Check sheet for the modelled part. Datum: model origin and axes. Units: mm. Face numbers are marked on the shaded views. A direction names the side the tool comes from. Coordinates: 2 decimals unless noted, no trailing zeros. Loops run counter-clockwise (first coordinate to the right, second up) from the corner with the lowest first, then second, coordinate; pieces in that order, holes last. Notation, with made-up numbers: M 52,-7.5 L 81,-7.5 A18 ccw 81,25.5 Z; hole C -33,65 d9. An arc over 180 degrees is marked long. Return JSON: item names as keys, results as strings.
from build123d import *

# Parameters (mm, degrees)
SKETCH1_R           = 9
BOSS_EXTRUDE1_DEPTH = 5
SKETCH2_R           = 3
SKETCH2_R_2         = 2
BOSS_EXTRUDE2_DEPTH = 6
CUT_EXTRUDE1_DEPTH  = 17.822603841
CUT_EXTRUDE2_DEPTH  = 3
CUT_EXTRUDE3_DEPTH  = 8


with BuildPart() as part:
    # Sketch1 → Boss-Extrude1 (new body)
    with BuildSketch(Plane.XY):
        Circle(SKETCH1_R)
    extrude(amount=BOSS_EXTRUDE1_DEPTH)

    # Sketch2 → Boss-Extrude2 (add)
    with BuildSketch(Plane.XY.offset(5)):
        Circle(SKETCH2_R)
        with Locations(Location((-7, 0, 0), (0, 0, 179.999350333))):
            Circle(SKETCH2_R_2)
    extrude(amount=BOSS_EXTRUDE2_DEPTH)

    # Sketch3 → Cut-Extrude1 (cut, through all)
    with BuildSketch(Plane.XY.offset(11)):
        Polygon((-1.616580754, 0), (-0.808290377, -1.4), (0.808290377, -1.4), (1.616580754, 0), (0.808290377, 1.4), (-0.808290377, 1.4), align=None)
    extrude(amount=-CUT_EXTRUDE1_DEPTH, mode=Mode.SUBTRACT)

    # Sketch4 → Cut-Extrude2 (cut)
    with BuildSketch(Plane(origin=(0, 0, 0), x_dir=(-1, 0, 0), z_dir=(0, 0, -1))):
        Polygon((-4.099186911, 0), (-2.049593456, -3.55), (2.049593456, -3.55), (4.099186911, 0), (2.049593456, 3.55), (-2.049593456, 3.55), align=None)
    extrude(amount=-CUT_EXTRUDE2_DEPTH, mode=Mode.SUBTRACT)

    # Sketch5 → Cut-Extrude3 (cut)
    with BuildSketch(Plane.XZ.offset(-3.55)):
        with BuildLine():
            Line((1, 1.756249669), (1, -1.040433474))
            Line((1, -1.040433474), (-1, -1.040433474))
            Line((-1, -1.040433474), (-1, 1.756249669))
            ThreePointArc((-1, 1.756249669), (0, 2.756249669), (1, 1.756249669))
        make_face()
    extrude(amount=-CUT_EXTRUDE3_DEPTH, mode=Mode.SUBTRACT)


solid = part.part
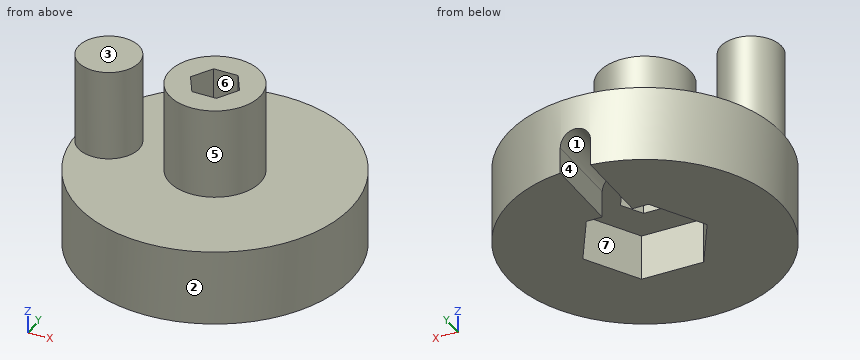
1) Scan lines: line 1 along Z through (x, y) = (3.5, -2); line 2 along Z through (x, y) = (-3.75, 0.5); line 3 along X through (y, z) = (1.5, 2). Record each from-to range of solid material in increasing order. Write a range as [from, to].
Answers:
{"line 1": "[0, 5]", "line 2": "[3, 5]", "line 3": "[-8.87, -3.23], [3.23, 8.87]"}
2) Go/stop test with flat-tipped pins: pin 1 Ø0.5 at (y, z) = (7, 0.5) entering from -X; pin 2 Ø1.4 at (y, z) = (5.5, 1) entering from +X; pin 3 Ø0.5 at (x, z) = (0, 6.5) entering from -Y; pin 4 Ø10 at (x, y) = (6.5, -1.5) entering from -Z. Record where each tip stops, or that it passes through.
Answers:
{"pin 1": "x = -5.95", "pin 2": "x = 7.61", "pin 3": "y = -3", "pin 4": "z = 0"}
3) Section check C-C on z = 3.25. Record the cut outline in (x, y), then the cut area to 3 significant figures.
Answers:
{"outline": "C 0,0 d18; hole M -1.62,0 L -0.81,-1.4 L 0.81,-1.4 L 1.62,0 L 0.81,1.4 L -0.81,1.4 Z", "area": "248 mm²"}
4) Section check B-B on x = 0. Record the cut outline in (y, z), then the cut area to 3 significant figures.
Answers:
{"outline": "M -9,0 L -3.55,0 L -3.55,3 L -1.4,3 L -1.4,11 L -3,11 L -3,5 L -9,5 Z; M 1.4,3 L 3.55,3 L 3.55,2.76 L 9,2.76 L 9,5 L 3,5 L 3,11 L 1.4,11 Z", "area": "67.3 mm²"}
5) Section check A-A on z = 7.5. Record the cut outline in (x, y), then the cut area to 3 significant figures.
Answers:
{"outline": "C -7,0 d4; C 0,0 d6; hole M -1.62,0 L -0.81,-1.4 L 0.81,-1.4 L 1.62,0 L 0.81,1.4 L -0.81,1.4 Z", "area": "34.1 mm²"}
6) Draft check along X on the marked faces 1, 2 and 3. Enter one of: +X half, -X half, draft (parallel to the pull), parting line (faces both ways), or undercut.
Answers:
{"face 1": "undercut", "face 2": "parting line", "face 3": "draft"}
7) Section check D-D on x = -7. Record the cut outline in (y, z), then the cut area to 3 significant figures.
Answers:
{"outline": "M -5.66,0 L 5.66,0 L 5.66,5 L 2,5 L 2,11 L -2,11 L -2,5 L -5.66,5 Z", "area": "80.6 mm²"}
8) Set-up check for the marked faces 4, 5, 6 and 7: record each of +Z, -Z, +X, -X, +Y, -Y from which the full face is reachable in a straight line by a thin tool's end or side.
Answers:
{"face 4": "-Z, +Y", "face 5": "+Z", "face 6": "+Z, -Z", "face 7": "-Z"}
